from build123d import *

# Parameters (mm, degrees)
SKETCH1_R               = 9
SKETCH1_R_2             = 5.9
BOSS_EXTRUDE1_DEPTH     = 19.8
CUT_EXTRUDE5_START      = 6.5
SKETCH3_R               = 7.65
CUT_EXTRUDE5_DEPTH      = 18.038054295
CUT_EXTRUDE6_DEPTH      = 27.707489752
CUT_EXTRUDE6_DEPTH_BACK = 7
SKETCH6_R               = 5.5
SKETCH7_R               = 12.932797278
CUT_EXTRUDE7_DEPTH      = 10


with BuildPart() as part:
    # Sketch1 → Boss-Extrude1 (new body)
    with BuildSketch(Plane(origin=(0, 0, 0), x_dir=(1, 0, 0), z_dir=(0, 1, 0))):
        with Locations(Location((0, 0, 0), (0, 0, 270))):
            Circle(SKETCH1_R)
        with Locations(Location((0, 0, 0), (0, 0, 270))):
            Circle(SKETCH1_R_2, mode=Mode.SUBTRACT)
    extrude(amount=-BOSS_EXTRUDE1_DEPTH)

    # Sketch3 → Cut-Extrude5 (cut, through all)
    with BuildSketch(Plane.XY.offset(CUT_EXTRUDE5_START)):
        with Locations((0, -8.4)):
            Circle(SKETCH3_R)
    extrude(amount=CUT_EXTRUDE5_DEPTH, mode=Mode.SUBTRACT)

    # Sketch6 → Cut-Extrude6 (cut, two sides: drawn at the far end of the back side and taken through both)
    with BuildSketch(Plane.XY.offset(6.5).offset(-CUT_EXTRUDE6_DEPTH_BACK)):
        with Locations(Location((0.145476138, -8.4, 0), (0, 0, 91.515662264))):
            Circle(SKETCH6_R)
    extrude(amount=CUT_EXTRUDE6_DEPTH + CUT_EXTRUDE6_DEPTH_BACK, mode=Mode.SUBTRACT)

    # Sketch7 → Cut-Extrude7 (cut)
    with BuildSketch(Plane(origin=(0, -13.8, 0), x_dir=(-1, 0, 0), z_dir=(0, -1, 0))):
        Circle(SKETCH7_R)
    extrude(amount=CUT_EXTRUDE7_DEPTH, mode=Mode.SUBTRACT)


solid = part.part
Geometry: final body of the model. Coordinates: model frame, mm. A direction names the side the tool comes from. Coordinates: 2 decimals unless noted, no trailing zeros. Order: outer loops, then holes, each group sorted by start corner. A loop starts at its lowest first (then second) coordinate and runs counter-clockwise, first axis right, second up.
1) Draft query along Y for faces 3 (the flat face through (4, -13.8, -5)), 4 (the flat face through (-2, -3, 6.5)), 5 (the flat face through (-6, 0, 2)). Return one class per face: released by +Y, released by -Y, zero draft, split by the parting line, or undercut.
Result sheet:
face 3: released by -Y
face 4: undercut
face 5: released by +Y
2) Set-up query: faces 1 (the cylindrical face through (0.259, -6.803, -5.894)), 2 (the cylindrical face through (-5.756, -13.438, 6.686)). Return all of +Z, -Z, +X, -X, +Y, -Y with unobstructed straight access to the full face (end or side cutting, diameter ignored); none if empty.
Result sheet:
face 1: +Y, -Y
face 2: +Z
3) Section C-C (x = 0). Return loops of the section in (y, z), then the cut area to 3 significant figures.
Result sheet:
outline: (-13.8, -9) - (0, -9) - (0, -5.9) - (-13.8, -5.9) - close; (-2.9, 5.9) - (0, 5.9) - (0, 9) - (-0.75, 9) - (-0.75, 6.5) - (-2.9, 6.5) - close
area: 46.4 mm2
4) Section B-B (x = -5). Return loops of the section in (y, z).
Result sheet:
outline: (-13.8, -7.48) - (0, -7.48) - (0, -3.13) - (-13.8, -3.13) - close; (-13.8, 3.13) - (-10.34, 3.13) - (-10.34, 6.5) - (-13.8, 6.5) - close; (-6.46, 3.13) - (0, 3.13) - (0, 7.48) - (-2.61, 7.48) - (-2.61, 6.5) - (-6.46, 6.5) - close
5) Section D-D (y = -1.5). Return loops of the section in (x, z).
Result sheet:
outline: (-3.3, 6.5) - (-3.3, 8.37) arc R9 ccw (long way) to (3.3, 8.37) - (3.3, 6.5) - close; hole circle Ø11.8 at (0, 0)
6) Section A-A (z = 0). Return loops of the section in (x, y), then the cut area to 3 significant figures.
Result sheet:
outline: (-9, -13.8) - (-5.9, -13.8) - (-5.9, 0) - (-9, 0) - close; (5.9, -13.8) - (9, -13.8) - (9, 0) - (5.9, 0) - close
area: 85.6 mm2
7) Ray query, probe 1 along X at (y, z) = (-2.75, 0); probe 2 along X at (y, z) = (-0.25, 1.25); probe 3 along Z at (x, y) = (-1.5, -0.5). Return the intervals inside material, ascending.
Result sheet:
probe 1: x = -9 to -5.9, 5.9 to 9
probe 2: x = -8.91 to -5.77, 5.77 to 8.91
probe 3: z = -8.87 to -5.71, 5.71 to 8.87
8) First-contact query: P1, Ø3, axis at y = -11, z = 3.5, coming from the -X side; P2, Ø1, axis at x = -4, y = -4.5, coming from the +Z side; P3, Ø1, axis at y = -2, z = -5, coming from the -X side. Flat tips, straight axial feed; report the tip coordinate or a pass-through.
Result sheet:
P1: stops at x = -8.77
P2: stops at z = 6.5
P3: stops at x = -7.79
